```python
from build123d import *

# Parameters (mm, degrees)
EXTRUDE_1_DEPTH     = 2
SKETCH_3_W          = 0.25
SKETCH_3_H          = 1.3
CUT_EXTRUDE_2_DEPTH = 1.2


with BuildPart() as part:
    # 草图1 → 凸台-拉伸1 (new body)
    with BuildSketch(Plane.XY):
        with BuildLine():
            Line((0, 0), (0, 0.5))
            Line((0, 0.5), (6.441160499, 0.162433082))
            ThreePointArc((6.441160499, 0.162433082), (6.961621967, -0.415597938), (7.539652987, 0.10486353))
            Line((7.539652987, 0.10486353), (9.48698058, 0.002808416))
            Line((9.48698058, 0.002808416), (9.476513389, -0.196917491))
            Line((9.476513389, -0.196917491), (7.701790537, -0.103908208))
            ThreePointArc((7.701790537, -0.103908208), (6.951154776, -0.615323845), (6.258088567, -0.028246994))
            Line((6.258088567, -0.028246994), (0.2, 0.289243975))
            Line((0.2, 0.289243975), (0.2, -0.2))
            Line((0.2, -0.2), (-1.8, -0.2))
            Line((-1.8, -0.2), (-1.8, -1.5))
            Line((-1.8, -1.5), (-2, -1.5))
            Line((-2, -1.5), (-2, 0))
            Line((-2, 0), (0, 0))
        make_face()
    extrude(amount=EXTRUDE_1_DEPTH)

    # 草图3 → 切除-拉伸2 (cut, through all)
    with BuildSketch(Plane(origin=(-1.8, 0, 0), x_dir=(0, 0, -1), z_dir=(1, 0, 0))):
        with Locations((-1.875, -0.85)):
            Rectangle(SKETCH_3_W, SKETCH_3_H)
        with Locations((-0.125, -0.85)):
            Rectangle(SKETCH_3_W, SKETCH_3_H)
    extrude(amount=-CUT_EXTRUDE_2_DEPTH, mode=Mode.SUBTRACT)


solid = part.part
```
Build history of the part. All positions in model axes, mm. A direction names the side the tool comes from. Round coordinates to 2 decimals unless told otherwise and drop trailing zeros. Write each loop counter-clockwise with the first axis right and the second up, starting at its lowest first coordinate (ties: lowest second). Pieces come first, ordered by that corner, then holes. Notation, with made-up numbers: (7.5, -12) - (20.5, -12) arc R18 ccw to (20.5, 23) - close; hole circle Ø7 at (-20, 8). An arc over 180 degrees is marked (long way). Answer as CSV lines item,"result".
Q1. Cut at A-A (y = -0.3). Write the cut outline in (x, z).
Report:
outline,"(-2, 0.25) - (-1.8, 0.25) - (-1.8, 1.75) - (-2, 1.75) - close; (6.38, 0) - (6.65, 0) - (6.65, 2) - (6.38, 2) - close; (7.33, 0) - (7.6, 0) - (7.6, 2) - (7.33, 2) - close"
Q2. Cut at B-B (z = 1.5). Write the cut outline in (x, y), and give its area (3 significant figures).
Report:
outline,"(-2, -1.5) - (-1.8, -1.5) - (-1.8, -0.2) - (0.2, -0.2) - (0.2, 0.29) - (6.26, -0.03) arc R0.75 ccw to (7.7, -0.1) - (9.48, -0.2) - (9.49, 0) - (7.54, 0.1) arc R0.55 cw to (6.44, 0.16) - (0, 0.5) - (0, 0) - (-2, 0) - close"
area,"2.77 mm^2"
Q3. Drill centre lines: probe 1 along X at (y, z) = (-0.25, 0.55); probe 2 along Y at (x, z) = (-0.5, 1.2); probe 3 along Y at (x, z) = (5.75, 1.9). Where is each one in solid material? Low to high. Write a range as [from, to].
Report:
probe 1,"x = [-2, -1.8], [6.35, 6.6], [7.38, 7.63]"
probe 2,"y = [-0.2, 0]"
probe 3,"y = [0, 0.2]"
Q4. Cut at C-C (y = -1.05). Write the cut outline in (x, z), and give its area (3 significant figures).
Report:
outline,"(-2, 0.25) - (-1.8, 0.25) - (-1.8, 1.75) - (-2, 1.75) - close"
area,"0.300 mm^2"
Q5. Cut at D-D (x = -1). Write the cut outline in (y, z).
Report:
outline,"(-0.2, 0) - (0, 0) - (0, 2) - (-0.2, 2) - close"
Q6. Tool access for faces 5 (the flat face through (-1.8, -1, 1)), 6 (the flat face through (-2, -1, 1)): list every direction of +Z, -Z, +X, -X, +Y, -Y with a clear straight run to the whole face (end or side of a thin tool).
Report:
face 5,"+Z, -Z, -Y"
face 6,"+Z, -Z, -X, +Y, -Y"
Q7. Pull direction X, two halves, no side cores. Call faces 1 (the flat face through (3.175, 0.334, 0.986)), 2 (the flat face through (-1, 0, 1)), 3 (the cylindrical face through (6.965, -0.616, 0.986)), 4 (the flat face through (3.27, 0.13, 0.99)): +X half, -X half, draft (parallel to the pull), parting line (faces both ways), or undercut.
Report:
face 1,"+X half"
face 2,"draft"
face 3,"undercut"
face 4,"undercut"
